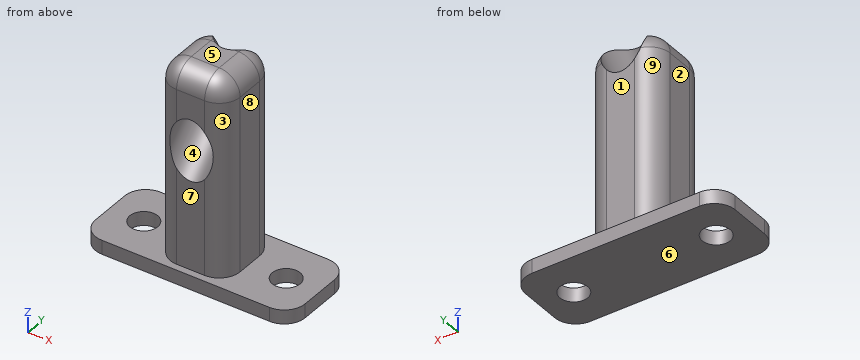
from build123d import *

# Parameters (mm, degrees)
F0_W     = 30
F0_H     = 12
F0_R     = 2
F0_W_2   = 10
F0_H_2   = 10
F1_DEPTH = 2
F2_DEPTH = 30
F3_R     = 3
F5_R     = 3.1
F6_DEPTH = 100


with BuildPart() as f1:
    # F0 (on Top) → F1 (new body)
    with BuildSketch(Plane.XY):
        Rectangle(F0_W, F0_H)
        with Locations((-10.187883, 0)):
            Circle(F0_R, mode=Mode.SUBTRACT)
        Rectangle(F0_W_2, F0_H_2, mode=Mode.SUBTRACT)
        with Locations((10.187883, 0)):
            Circle(F0_R, mode=Mode.SUBTRACT)
        Rectangle(F0_W_2, F0_H_2)
    extrude(amount=F1_DEPTH)

    # F0 (on Top) → F2 (join)
    with BuildSketch(Plane.XY):
        Rectangle(F0_W_2, F0_H_2)
    extrude(amount=F2_DEPTH)

    # F3
    f3_edges = [f1.edges().sort_by_distance(p)[0] for p in [
        (-15, -6, 1),
        (-5, -5, 16),
        (5, -5, 16),
        (5, 5, 16),
        (15, -6, 1),
        (15, 6, 1),
        (-5, 5, 16),
        (-15, 6, 1),
        (5, 0, 30),
        (0, 5, 30),
        (-5, 0, 30),
        (0, -5, 30),
    ]]
    fillet(f3_edges, radius=F3_R)

    # F5 (on face) → F6 (cut)
    with BuildSketch(Plane(origin=(0, -3, -3), x_dir=(1, 0, 0), z_dir=(0, -0.707107, -0.707107))):
        with Locations((0, 17.014893)):
            Circle(F5_R)
    extrude(amount=-F6_DEPTH, mode=Mode.SUBTRACT)


solid = f1.part
Verification items for the finished model (mm, model axes). Face numbers are marked on the shaded views. A direction names the side the tool comes from. Round coordinates to 2 decimals unless told otherwise and drop trailing zeros. Loops run counter-clockwise (first coordinate to the right, second up) from the corner with the lowest first, then second, coordinate; pieces in that order, holes last. Notation, with made-up numbers: (-16, -26.5) - (8, -26.5) arc R14 cw to (8, -17.5) - close; hole circle Ø10 at (17.5, -10). An arc over 180 degrees is marked (long way). Use a Markdown table: item, result. Add a question column.
1. Gauge pin test, flat ends, axial feed: pin 1 (2 mm diameter, centred on x = -1, z = 7, fed in from -Y); pin 2 (1.2 mm diameter, centred on y = -1, z = 13.5, fed in from -X); pin 3 (1.5 mm diameter, centred on x = 1.5, z = 23, fed in from +Y). Record the tip position at first contact, or that the pin passes through.
2. Thickness scan on probe 1 along X at (y, z) = (-2, 10); probe 2 along Z at (x, y) = (-1, -1.25); probe 3 along Z at (x, y) = (11.75, -5.5). Record the ranges inside material, lowest first. Write a range as [from, to].
3. Access from +Z, -Z, +X, -X, +Y, -Y to the whole of each face (thin tool, end or side, straight path). Record for the marked faces 5, 6, 7, 8 and 9.
4. Section check C-C, the plane x = -6.75. Record the boundary of the cut face in (y, z), plus the area to 3 significant figures.
5. Release check for a two-part mould opening along X. For the marked faces 1, 2, 3 and 4 record: released by +X, released by -X, zero draft, split by the parting line, or undercut.
6. Section check A-A, the plane z = 8.5. Record the boundary of the cut face in (x, y), plus the area to 3 significant figures.
7. Section check B-B, the plane y = 0. Give the number of separate pieces and of enclosed holes in the cut face, plus the area to 3 significant figures.
Checks:
| question | item | result |
|---|---|---|
| 1 | pin 1 | stops at y = -5 |
| 1 | pin 2 | stops at x = -5 |
| 1 | pin 3 | stops at y = 5 |
| 2 | probe 1 | x = [-5, 5] |
| 2 | probe 2 | z = [0, 18.66], [26.96, 30] |
| 2 | probe 3 | z = [0, 2] |
| 3 | face 5 | +Z, +X, -X, +Y, -Y |
| 3 | face 6 | -Z, +X, -X, +Y, -Y |
| 3 | face 7 | +Z, +X, -X, -Y |
| 3 | face 8 | +Z, +X, +Y, -Y |
| 3 | face 9 | +Z, -X, +Y |
| 4 | outline | (-6, 0) - (6, 0) - (6, 2) - (-6, 2) - close |
| 4 | area | 24.0 mm^2 |
| 5 | face 1 | zero draft |
| 5 | face 2 | released by -X |
| 5 | face 3 | released by +X |
| 5 | face 4 | undercut |
| 6 | outline | (-5, -2) arc R3 ccw to (-2, -5) - (2, -5) arc R3 ccw to (5, -2) - (5, 2) arc R3 ccw to (2, 5) - (-2, 5) arc R3 ccw to (-5, 2) - close |
| 6 | area | 92.3 mm^2 |
| 7 | separate pieces | 3 |
| 7 | enclosed holes | 1 |
| 7 | area | 277 mm^2 |
